The model under review builds one solid part; all positions refer to its coordinate system, in mm. Round coordinates to 2 decimals unless told otherwise and drop trailing zeros. Loops run counter-clockwise (first coordinate to the right, second up) from the corner with the lowest first, then second, coordinate; pieces in that order, holes last. Notation, with made-up numbers: M 7.25,-37.75 L 34.25,-37.75 A15 cw 34.25,-29.75 Z; hole C 45.5,40 d3. An arc over 180 degrees is marked long. Answer in a Markdown table with one row per item. Add a question column.
from build123d import *

# Parameters (mm, degrees)
SKETCH1_R           = 1.5
BOSS_EXTRUDE1_DEPTH = 2
CUT_EXTRUDE1_DEPTH  = 197.459257863
CHAMFER1_SIZE       = 2


with BuildPart() as part:
    # Sketch1 → Boss-Extrude1 (new body)
    with BuildSketch(Plane.XY):
        with BuildLine():
            Line((102.318351238, 102.318351238), (113.419927702, 113.419927702))
            ThreePointArc((113.419927702, 113.419927702), (160.4, 0), (113.419927702, -113.419927702))
            Line((113.419927702, -113.419927702), (102.318351238, -102.318351238))
            ThreePointArc((102.318351238, -102.318351238), (144.7, 0), (102.318351238, 102.318351238))
        make_face()
        with Locations((121.321245866, 98.702154493)):
            Circle(SKETCH1_R, mode=Mode.SUBTRACT)
        with Locations((143.451847555, 62.309930452)):
            Circle(SKETCH1_R, mode=Mode.SUBTRACT)
        with Locations((154.94328196, 21.296463919)):
            Circle(SKETCH1_R, mode=Mode.SUBTRACT)
        with Locations((154.94328196, -21.296463919)):
            Circle(SKETCH1_R, mode=Mode.SUBTRACT)
        with Locations((143.451847555, -62.309930452)):
            Circle(SKETCH1_R, mode=Mode.SUBTRACT)
        with Locations((121.321245866, -98.702154493)):
            Circle(SKETCH1_R, mode=Mode.SUBTRACT)
        with Locations(Location((127.774091267, 90.192802379, 0), (0, 0, 180))):
            Circle(SKETCH1_R, mode=Mode.SUBTRACT)
        with Locations(Location((147.369608219, 52.375171344, 0), (0, 0, 180))):
            Circle(SKETCH1_R, mode=Mode.SUBTRACT)
        with Locations(Location((153.128751314, 31.820520441, 0), (0, 0, 180))):
            Circle(SKETCH1_R, mode=Mode.SUBTRACT)
        with Locations(Location((156.035395501, 10.67311345, 0), (0, 0, 180))):
            Circle(SKETCH1_R, mode=Mode.SUBTRACT)
        with Locations(Location((127.774091267, -90.192802379, 0), (0, 0, 180))):
            Circle(SKETCH1_R, mode=Mode.SUBTRACT)
        with Locations(Location((147.369608219, -52.375171344, 0), (0, 0, 180))):
            Circle(SKETCH1_R, mode=Mode.SUBTRACT)
        with Locations(Location((153.128751314, -31.820520441, 0), (0, 0, 180))):
            Circle(SKETCH1_R, mode=Mode.SUBTRACT)
        with Locations(Location((156.035395501, -10.67311345, 0), (0, 0, 180))):
            Circle(SKETCH1_R, mode=Mode.SUBTRACT)
        with Locations((138.865248158, 71.954171901)):
            Circle(SKETCH1_R, mode=Mode.SUBTRACT)
        with Locations((114.302744813, 106.751311599)):
            Circle(SKETCH1_R, mode=Mode.SUBTRACT)
        with Locations((138.865248158, -71.954171901)):
            Circle(SKETCH1_R, mode=Mode.SUBTRACT)
        with Locations((114.302744813, -106.751311599)):
            Circle(SKETCH1_R, mode=Mode.SUBTRACT)
    extrude(amount=BOSS_EXTRUDE1_DEPTH)

    # Sketch2 → Cut-Extrude1 (cut, through all)
    with BuildSketch(Plane.XY.offset(2)):
        Polygon((117.10590357, 116.893771535), (92.696291985, 92.484159951), (81.614099529, 103.566352407), (106.023711114, 127.975963992), align=None)
        Polygon((94.953094668, -94.740962634), (127.588403443, -127.376271408), (106.110382849, -148.854292002), (73.475074075, -116.218983227), align=None)
    extrude(amount=-CUT_EXTRUDE1_DEPTH, mode=Mode.SUBTRACT)

    # Chamfer1
    chamfer1_edges = [part.edges().sort_by_distance(p)[0] for p in [
        (119.821245866, 98.702154493, 2),
        (141.951847555, 62.309930452, 2),
        (153.44328196, 21.296463919, 2),
        (153.44328196, -21.296463919, 2),
        (141.951847555, -62.309930452, 2),
        (119.821245866, -98.702154493, 2),
        (129.274091267, 90.192802379, 2),
        (148.869608219, 52.375171344, 2),
        (154.628751314, 31.820520441, 2),
        (157.535395501, 10.67311345, 2),
        (129.274091267, -90.192802379, 2),
        (148.869608219, -52.375171344, 2),
        (154.628751314, -31.820520441, 2),
        (157.535395501, -10.67311345, 2),
        (112.802744813, 106.751311599, 2),
        (137.365248158, 71.954171901, 2),
        (137.365248158, -71.954171901, 2),
        (112.802744813, -106.751311599, 2),
    ]]
    chamfer(chamfer1_edges, length=CHAMFER1_SIZE - 0.0001)  # a hair under: the kernel refuses the full size


solid = part.part
1. Take a section at B-B, the plane y = -1. State the section outline as (x, z) points.
2. Take a section at A-A, the plane z = 0.8. State how many separate pieces and enclosed holes the cut face has, and give its area (3 significant figures).
3. To check wall thickness, follow probe 1 along Y at (x, z) = (115, 1.6); probe 2 along Y at (x, z) = (128.5, 1.7); probe 3 along X at (y, z) = (61, 1.1). State the ranges of each line that lie inside material, in increasing order.
4. For pin 1 Ø2.5 at (x, y) = (127.77, 90.19) entering from -Z; pin 2 Ø1 at (x, z) = (119, 1) entering from -Y; pin 3 Ø5 at (x, y) = (127.77, -90.19) entering from +Z; pin 4 Ø3.5 at (x, y) = (114.3, 106.75) entering from +Z, all flat-tipped, find the tip position at first contact; note any pin that passes through.
5. Take a section at C-C, the plane y = -80.5. State the section outline as (x, z) points.
Check sheet entries:
| question | item | result |
|---|---|---|
| 1 | outline | M 144.7,0 L 160.4,0 L 160.4,2 L 144.7,2 Z |
| 2 | separate pieces | 1 |
| 2 | enclosed holes | 18 |
| 2 | area | 3,460 mm^2 |
| 3 | probe 1 | y = -111.82 to -109.77, -103.73 to -87.82, 87.82 to 103.73, 109.77 to 111.82 |
| 3 | probe 2 | y = -96 to -93.31, -87.08 to -66.53, 66.53 to 87.08, 93.31 to 96 |
| 3 | probe 3 | x = 131.21 to 141.21, 145.7 to 148.35 |
| 4 | pin 1 | passes through |
| 4 | pin 2 | stops at y = -108.1 |
| 4 | pin 3 | stops at z = 1.01 |
| 4 | pin 4 | stops at z = 0.25 |
| 5 | outline | M 120.24,0 L 138.74,0 L 138.74,2 L 120.24,2 Z |
